from build123d import *

# Parameters (mm, degrees)
SKETCH2_R               = 12.7
SKETCH2_R_2             = 11.7
CUT_EXTRUDE1_DEPTH      = 1065.529727188
CUT_EXTRUDE1_DEPTH_BACK = 1065.529727188
SKETCH3_R               = 3.3782
CUT_EXTRUDE2_DEPTH      = 1065.529727283
CUT_EXTRUDE2_DEPTH_BACK = 1065.529727283
SKETCH4_R               = 3.3782


with BuildPart() as part:
    # Sweep-Thin1: sweep along a path in Sketch1
    with BuildLine(Plane(origin=(0, 0, 0), x_dir=(1, 0, 0), z_dir=(0, 1, 0))) as sweep_thin1_path:
        Line((-1016, 304.8), (-76.2, 304.8))
        ThreePointArc((-76.2, 304.8), (-22.318463274, 282.481536726), (0, 228.6))
        Line((0, 228.6), (0, -228.6))
        ThreePointArc((0, -228.6), (-22.318463274, -282.481536726), (-76.2, -304.8))
        Line((-76.2, -304.8), (-1016, -304.8))
    # Sketch2 → Sweep-Thin1 (sweep)
    with BuildSketch(Plane(origin=(-1016, 0, 0), x_dir=(0, 0, -1), z_dir=(1, 0, 0))):
        with Locations((304.8, 0)):
            Circle(SKETCH2_R)
        with Locations((304.8, 0)):
            Circle(SKETCH2_R_2, mode=Mode.SUBTRACT)
    sweep(path=sweep_thin1_path.line)

    # Sketch3 → Cut-Extrude1 (cut, two sides: drawn at the far end of the back side and taken through both)
    with BuildSketch(Plane.XY.offset(-CUT_EXTRUDE1_DEPTH_BACK)):
        with Locations((-1000.76, 0)):
            Circle(SKETCH3_R)
    extrude(amount=CUT_EXTRUDE1_DEPTH + CUT_EXTRUDE1_DEPTH_BACK, mode=Mode.SUBTRACT)

    # Sketch4 → Cut-Extrude2 (cut, two sides: drawn at the far end of the back side and taken through both)
    with BuildSketch(Plane.XY.offset(-CUT_EXTRUDE2_DEPTH_BACK)):
        with Locations((-848.36, 0)):
            Circle(SKETCH4_R)
    extrude(amount=CUT_EXTRUDE2_DEPTH + CUT_EXTRUDE2_DEPTH_BACK, mode=Mode.SUBTRACT)


solid = part.part
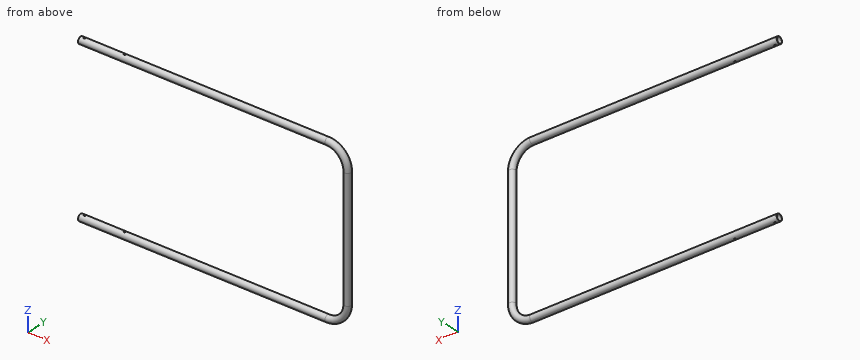
Design review of the part built by this model. Coordinates are the model's own, in mm. Give positions to 0.01 mm unless a question says otherwise; leave off trailing zeros. Order: outer loops, then holes, each group sorted by start corner. A loop starts at its lowest first (then second) coordinate and runs counter-clockwise, first axis right, second up. Notation, with made-up numbers: (49.5, -38.5) - (95.5, -38.5) arc R22 ccw to (95.5, -9.5) - close; hole circle Ø4 at (-7, -15). An arc over 180 degrees is marked (long way). Write item = value, one per line. Start each with the question number.
Q1. We need section A-A on x = -706. State the section outline as (y, z) points.
Q2. To check wall thickness, follow L1, parallel to Z at x = -214, y = 1; L2, parallel to Y at x = -275, z = 304.8; L3, parallel to Z at x = -718.5, y = -1.5. State the ranges of each line that lie inside material, in increasing order. Write a range as from..to.
Q3. Clearance check with flat-ended pins moving along their axes: pin 1 Ø6 at (x, y) = (-848.36, 0) entering from -Z; pin 2 Ø5 at (y, z) = (6.5, -21) entering from +X; pin 3 Ø2 at (x, y) = (-643, 2) entering from +Z; pin 4 Ø5 at (x, y) = (-597.5, 3.5) entering from -Z. State where each tip first meets the part, or that it passes through.
Q4. We need section B-B on z = -1.5. State the section outline as (x, y) points.
Working result:
q1.outline = circle Ø25.4 at (0, -304.8); circle Ø25.4 at (0, 304.8); hole circle Ø23.4 at (0, -304.8); hole circle Ø23.4 at (0, 304.8)
q2.L1 = -317.46..-316.46, -293.14..-292.14, 292.14..293.14, 316.46..317.46
q2.L2 = -12.7..-11.7, 11.7..12.7
q2.L3 = -317.41..-316.4, -293.2..-292.19, 292.19..293.2, 316.4..317.41
q3.pin_1 = through
q3.pin_2 = 12.05
q3.pin_3 = 317.46
q3.pin_4 = -317.46
q4.outline = circle Ø25.4 at (0, 0); hole circle Ø23.4 at (0, 0)
